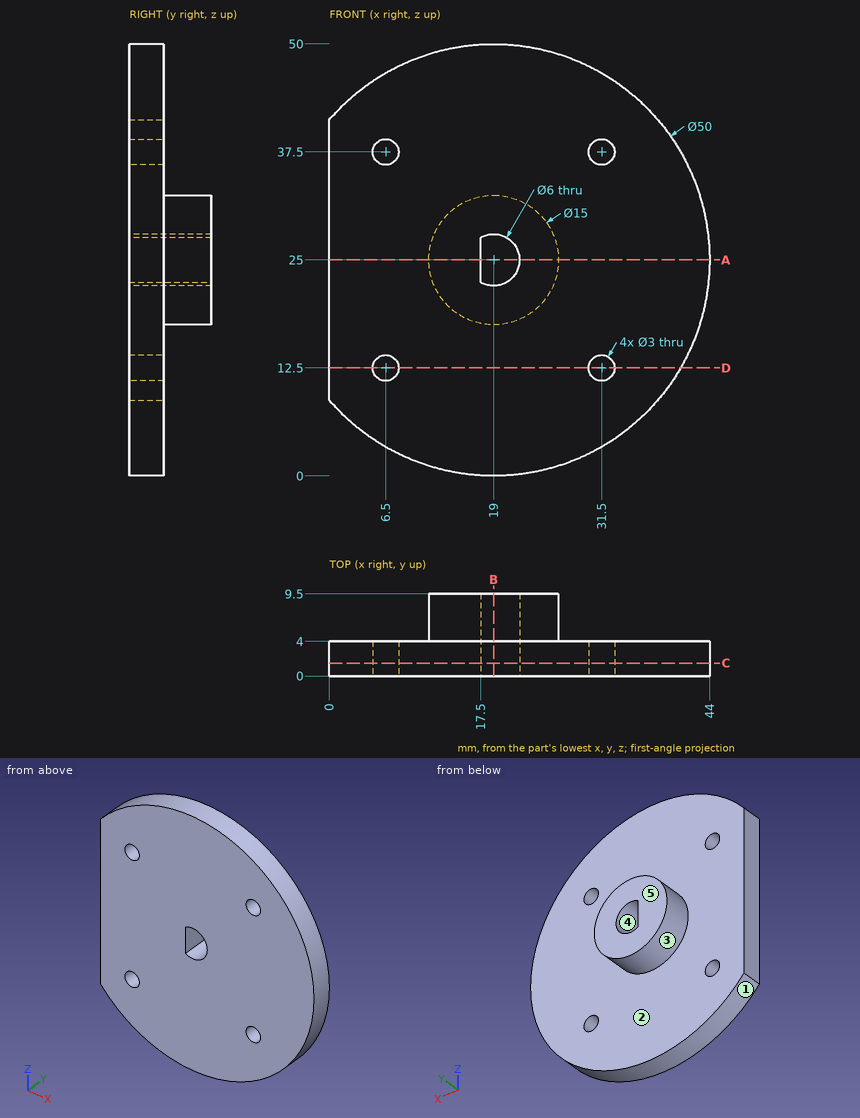
Study the drawing (mm; zero at the part's minimum x, y, z) and answer. A direction names the side the tool comes from. Coordinates: 2 decimals unless noted, no trailing zeros. Loops run counter-clockwise (first coordinate to the right, second up) from the corner with the lowest first, then second, coordinate; pieces in that order, holes last. Notation, with made-up numbers: (20.25, -14) -> (24.25, -14) arc R21 cw to (24.25, -1) -> close; hole circle Ø8 at (28.5, 12.25). An arc over 180 degrees is marked (long way). Answer in a Markdown table with one row per item. Add a question column.
1. For the marked faces 1 and 2, determine the directions among +Z, -Z, +X, -X, +Y, -Y from which every point of the face is accessible in a straight line to the end or side of a thin tool.
2. The part is cut by section A-A, the plane z = 25. Write down the section's boundary in (x, y).
3. The part is cut by section B-B, the plane x = 19. Write down the section's boundary in (y, z), then the cut area to 4 significant figures.
4. The part is cut by section C-C, the plane y = 1.5. Write down the section's boundary in (x, z), then the cut area to 3 significant figures.
5. The part is cut by section D-D, the plane z = 12.5. Write down the section's boundary in (x, y).
6. Consider line 1 (X direction, y = 2.45, z = 12.5); line 2 (X direction, y = 2.5, z = 12); line 3 (Y direction, x = 35, z = 19). Determine where each line is inside the solid, lowest interval first. Write a range as [from, to].
7. Flat-ended cylindrical pins translate along their axes: P1, Ø1.6, axis at y = 5.5, z = 25, coming from the +X side; P2, Ø2, axis at x = 21, y = 8, coming from the -Z side; P3, Ø3, axis at y = 3.5, z = 45, coming from the +X side. Find the tip coordinate at first contact, or state that the pin passes through.
8. Determine the mould class of the marked faces 3, 4 and 5 for opening direction X: +X half, -X half, draft (parallel to the pull), parting line (faces both ways), or undercut.
Answer below:
| question | item | result |
|---|---|---|
| 1 | face 1 | +Y, -Y |
| 1 | face 2 | +Y |
| 2 | outline | (0, 0) -> (17.5, 0) -> (17.5, 9.5) -> (11.5, 9.5) -> (11.5, 4) -> (0, 4) -> close; (22, 0) -> (44, 0) -> (44, 4) -> (26.5, 4) -> (26.5, 9.5) -> (22, 9.5) -> close |
| 3 | outline | (0, 0) -> (4, 0) -> (4, 17.5) -> (9.5, 17.5) -> (9.5, 22) -> (0, 22) -> close; (0, 28) -> (9.5, 28) -> (9.5, 32.5) -> (4, 32.5) -> (4, 50) -> (0, 50) -> close |
| 3 | area | 225.5 mm2 |
| 4 | outline | (0, 8.75) arc R25 ccw (long way) to (0, 41.25) -> close; hole circle Ø3 at (6.5, 12.5); hole circle Ø3 at (6.5, 37.5); hole (17.5, 22.4) arc R3 ccw (long way) to (17.5, 27.6) -> close; hole circle Ø3 at (31.5, 12.5); hole circle Ø3 at (31.5, 37.5) |
| 4 | area | 1,780 mm2 |
| 5 | outline | (0, 0) -> (5, 0) -> (5, 4) -> (0, 4) -> close; (8, 0) -> (30, 0) -> (30, 4) -> (8, 4) -> close; (33, 0) -> (40.65, 0) -> (40.65, 4) -> (33, 4) -> close |
| 6 | line 1 | [0, 5], [8, 30], [33, 40.65] |
| 6 | line 2 | [0, 5.09], [7.91, 30.09], [32.91, 40.35] |
| 6 | line 3 | [0, 4] |
| 7 | P1 | x = 26.5 |
| 7 | P2 | z = 17.57 |
| 7 | P3 | x = 35.82 |
| 8 | face 3 | parting line |
| 8 | face 4 | undercut |
| 8 | face 5 | draft |
